```python
from build123d import *

# Parameters (mm, degrees)
SKETCH1_W           = 55
SKETCH1_H           = 28.5
BOSS_EXTRUDE1_DEPTH = 2
SKETCH2_W           = 8
SKETCH2_H           = 7
BOSS_EXTRUDE2_DEPTH = 3
FILLET2_R           = 1
SHELL2_START        = -27.3
SHELL2_OUTLINE_W    = 28.1
SHELL2_OUTLINE_H    = 3.6
SHELL2_DEPTH        = 54.6
SHELL2_START_2      = 22.7
SHELL2_2_DEPTH      = 6.8
SHELL2_3_OUTLINE_W  = 7.6
SHELL2_3_OUTLINE_H  = 0.4
SHELL2_3_DEPTH      = 4.6
SKETCH3_R           = 0.5
BOSS_EXTRUDE3_DEPTH = 6


# Read off the part's stored shape, not the designer's step: Shell2
with BuildPart() as part:
    # Sketch1 → Boss-Extrude1 (new, symmetric)
    with BuildSketch(Plane(origin=(0, 0, 0), x_dir=(0, 1, 0), z_dir=(0, 0, 1))):
        Rectangle(SKETCH1_W, SKETCH1_H)
    extrude(amount=BOSS_EXTRUDE1_DEPTH, both=True)

    # Sketch2 → Boss-Extrude2 (add)
    with BuildSketch(Plane.XY.offset(2)):
        with Locations((-0.123519145, 26)):
            Rectangle(SKETCH2_W, SKETCH2_H)
    extrude(amount=BOSS_EXTRUDE2_DEPTH)

    # Fillet2
    fillet2_edges = [part.edges().sort_by_distance(p)[0] for p in [
        (3.876480855, 26, 5),
        (-4.123519145, 26, 5),
    ]]
    fillet(fillet2_edges, radius=FILLET2_R)

    # Shell2 outline → Shell2 (cut)
    with BuildSketch(Plane(origin=(0, 0, 0), x_dir=(1, 0, 0), z_dir=(0, 1, 0)).offset(SHELL2_START)):
        Rectangle(SHELL2_OUTLINE_W, SHELL2_OUTLINE_H)
    extrude(amount=SHELL2_DEPTH, mode=Mode.SUBTRACT)

    # Shell2 2 outline → Shell2 2 (cut)
    with BuildSketch(Plane(origin=(0, 0, 0), x_dir=(1, 0, 0), z_dir=(0, 1, 0)).offset(SHELL2_START_2)):
        with BuildLine():
            Line((3.676480855, -4), (3.676480855, -2.2))
            Line((3.676480855, -2.2), (-3.923519145, -2.2))
            Line((-3.923519145, -2.2), (-3.923519145, -4))
            ThreePointArc((-3.923519145, -4), (-3.68920457, -4.565685425), (-3.123519145, -4.8))
            Line((-3.123519145, -4.8), (2.876480855, -4.8))
            ThreePointArc((2.876480855, -4.8), (3.44216628, -4.565685425), (3.676480855, -4))
        make_face()
    extrude(amount=SHELL2_2_DEPTH, mode=Mode.SUBTRACT)

    # Shell2 3 outline → Shell2 3 (cut)
    with BuildSketch(Plane(origin=(0, 0, 0), x_dir=(1, 0, 0), z_dir=(0, 1, 0)).offset(SHELL2_START_2)):
        with Locations((-0.123519145, -2)):
            Rectangle(SHELL2_3_OUTLINE_W, SHELL2_3_OUTLINE_H)
    extrude(amount=SHELL2_3_DEPTH, mode=Mode.SUBTRACT)

    # Sketch3 → Boss-Extrude3 (add)
    with BuildSketch(Plane(origin=(0, 0, -2), x_dir=(1, 0, 0), z_dir=(0, 0, -1))):
        with Locations(Location((12.75, 23, 0), (0, 0, 180))):
            Circle(SKETCH3_R)
        with Locations(Location((12.75, 20.5, 0), (0, 0, 180))):
            Circle(SKETCH3_R)
        with Locations(Location((12.75, 18, 0), (0, 0, 180))):
            Circle(SKETCH3_R)
        with Locations(Location((12.75, 15.5, 0), (0, 0, 180))):
            Circle(SKETCH3_R)
        with Locations(Location((12.75, 13, 0), (0, 0, 180))):
            Circle(SKETCH3_R)
        with Locations(Location((12.75, 10.5, 0), (0, 0, 180))):
            Circle(SKETCH3_R)
        with Locations(Location((12.75, 8, 0), (0, 0, 180))):
            Circle(SKETCH3_R)
        with Locations(Location((12.75, 5.5, 0), (0, 0, 180))):
            Circle(SKETCH3_R)
        with Locations(Location((12.75, 3, 0), (0, 0, 180))):
            Circle(SKETCH3_R)
        with Locations(Location((12.75, 0.5, 0), (0, 0, 180))):
            Circle(SKETCH3_R)
        with Locations(Location((12.75, -2, 0), (0, 0, 180))):
            Circle(SKETCH3_R)
        with Locations(Location((12.75, -4.5, 0), (0, 0, 180))):
            Circle(SKETCH3_R)
        with Locations(Location((12.75, -7, 0), (0, 0, 180))):
            Circle(SKETCH3_R)
        with Locations(Location((12.75, -9.5, 0), (0, 0, 180))):
            Circle(SKETCH3_R)
        with Locations(Location((12.75, -12, 0), (0, 0, 180))):
            Circle(SKETCH3_R)
        with Locations(Location((12.75, -14.5, 0), (0, 0, 180))):
            Circle(SKETCH3_R)
        with Locations(Location((12.75, -17, 0), (0, 0, 180))):
            Circle(SKETCH3_R)
        with Locations(Location((12.75, -19.5, 0), (0, 0, 180))):
            Circle(SKETCH3_R)
        with Locations(Location((12.75, -22, 0), (0, 0, 180))):
            Circle(SKETCH3_R)
    boss_extrude3 = extrude(amount=BOSS_EXTRUDE3_DEPTH)

    # Mirror1: Boss-Extrude3 across plane
    add(boss_extrude3.mirror(Plane(origin=(0, 0, 0), x_dir=(0, 0, 1), z_dir=(1, 0, 0))))


solid = part.part
```
Geometry check sheet. Reference: the model listing, model coordinates, mm. A direction names the side the tool comes from. Round coordinates to 2 decimals unless told otherwise and drop trailing zeros. Order: outer loops, then holes, each group sorted by start corner. A loop starts at its lowest first (then second) coordinate and runs counter-clockwise, first axis right, second up. Notation, with made-up numbers: (6, 10.25) - (29, 10.25) arc R27 cw to (29, 46.25) - close; hole circle Ø11 at (-20, -17.75). An arc over 180 degrees is marked (long way). Use a Markdown table: item, result. Add a question column.
(1) Sectioned sample at C-C, the plane x = 1. Enter the section's corners in (y, z).
(2) Depth check by flat-ended pin: pin 1 (0.6 mm diameter, centred on y = 27, z = 3, fed in from -X); pin 2 (3 mm diameter, centred on x = 1, y = 27, fed in from -Z); pin 3 (0.9 mm diameter, centred on x = 1, z = 3, fed in from +Y). Enter the tip coordinate at first touch or a pass-through.
(3) Sectioned sample at D-D, the plane z = 3. Enter the section's corners in (x, y), and give its area (3 significant figures).
(4) Sectioned sample at B-B, the plane z = -1.25. Enter the section's corners in (x, y), and give its area (3 significant figures).
(5) Release check for a two-part mould opening along X. For faces 4 (the flat face through (0, 22.7, 3)), 5 (the cylindrical face through (-3.84, 26.05, 4.7)), 6 (the flat face through (3.876, 26, 3)), 7 (the cylindrical face through (12.815, 19.996, -4.958)) record: pulls with the +X half, pulls with the -X half, needs draft (parallel to the pull), parting line crosses it, or undercut.
(6) Material ranges on line 1 along Z through (x, y) = (-1.75, -18.5); line 2 along X through (y, z) = (1.5, 0); line 3 along Y through (x, z) = (5.5, 1), recorded low to high. Write a range as [from, to].
(7) Tool access check on faces 1 (the cylindrical face through (-12.519, -13.444, -4.958)), 2 (the flat face through (0, 22.5, 3)), 3 (the flat face through (13, 12, -8)). Record the directions out of +Z, -Z, +X, -X, +Y, -Y that give a thin tool (end or side, any length) a straight path to the whole face; none if there is none.
(8) Sectioned sample at A-A, the plane x = 9.5. Enter the section's corners in (y, z).
Answers below:
| question | item | result |
|---|---|---|
| 1 | outline | (-27.5, -2) - (27.5, -2) - (27.5, 2) - (29.5, 2) - (29.5, 2.2) - (27.3, 2.2) - (27.3, -1.8) - (-27.3, -1.8) - (-27.3, 1.8) - (22.7, 1.8) - (22.7, 4.8) - (29.5, 4.8) - (29.5, 5) - (22.5, 5) - (22.5, 2) - (-27.5, 2) - close |
| 2 | pin 1 | x = -4.12 |
| 2 | pin 2 | z = -2 |
| 2 | pin 3 | y = 22.7 |
| 3 | outline | (-4.12, 22.5) - (3.88, 22.5) - (3.88, 29.5) - (3.68, 29.5) - (3.68, 22.7) - (-3.92, 22.7) - (-3.92, 29.5) - (-4.12, 29.5) - close |
| 3 | area | 4.32 mm² |
| 4 | outline | (-14.25, -27.5) - (14.25, -27.5) - (14.25, 27.5) - (-14.25, 27.5) - close; hole (-14.05, -27.3) - (14.05, -27.3) - (14.05, 27.3) - (-14.05, 27.3) - close |
| 4 | area | 33.2 mm² |
| 5 | face 4 | undercut |
| 5 | face 5 | pulls with the -X half |
| 5 | face 6 | pulls with the +X half |
| 5 | face 7 | undercut |
| 6 | line 1 | [-2, -1.8], [1.8, 2] |
| 6 | line 2 | [-14.25, -14.05], [14.05, 14.25] |
| 6 | line 3 | [-27.5, -27.3], [27.3, 27.5] |
| 7 | face 1 | -Z |
| 7 | face 2 | +Z, +X, -X, -Y |
| 7 | face 3 | -Z, +X, -X, +Y, -Y |
| 8 | outline | (-27.5, -2) - (27.5, -2) - (27.5, 2) - (-27.5, 2) - close; hole (-27.3, -1.8) - (27.3, -1.8) - (27.3, 1.8) - (-27.3, 1.8) - close |
